Work out the finished part from the listing and answer in its coordinate system (mm). A direction names the side the tool comes from. Give positions to 0.01 mm unless a question says otherwise; leave off trailing zeros. Loops run counter-clockwise (first coordinate to the right, second up) from the corner with the lowest first, then second, coordinate; pieces in that order, holes last. Notation, with made-up numbers: (9, -25.75) - (36, -25.75) arc R25 ccw to (36, -12.75) - close; hole circle Ø11 at (-18.5, 69.5). An arc over 180 degrees is marked (long way). One line per question, with ' | ' between items. Start each with the question number.
1. Section C-C (y = 6.25) is taken. Determine the outline of the cut face in (x, z), plus the area to 3 significant figures.
2. Section B-B (x = 52) is taken. Determine the outline of the cut face in (y, z).
3. Find the intervals of material crossed by line 1 (Y direction, x = 34.5, z = 1.75); line 2 (X direction, y = 5, z = 12.75); line 3 (Y direction, x = 26.5, z = 7.5), in increasing order.
4. Which of the six approach directions +Z, -Z, +X, -X, +Y, -Y give full straight-line access (tool end or side, diameter ignored) to faces 1 (the face through (31, 21.971, 13)), 2 (the face through (1.651, 11, 6)), 3 (the face through (1.604, 20.45, 13.282)), 4 (the face through (31, 11.915, 5)), 5 (the face through (2.664, 11, 8))?
5. Each of these flat-tipped pins is pushed along its axis until it touches: pin 1 (3.5 mm diameter, centred on x = 34.5, z = 7.5, fed in from -Y); pin 2 (3 mm diameter, centred on y = 7, z = 9, fed in from -X); pin 3 (4 mm diameter, centred on x = 35, y = 11, fed in from +Z). Where does it stop, or does it pass through?
Autodesk Inventor part; units mm, degrees
ref_plane "YZ Plane" through (0, 0, 0) normal (1, 0, 0) x (0, 1, 0)
ref_plane "XZ Plane" through (0, 0, 0) normal (0, 1, 0) x (-1, 0, 0)
ref_plane "XY Plane" through (0, 0, 0) normal (0, 0, 1) x (1, 0, 0)
sketch "Sketch1" plane through (0, 0, 0) normal (0, 0, 1) x (1, 0, 0)
  line L0 (0, 0) -> (60.7568, 0)
  line L1 (60.7568, 0) -> (60.7568, 21.971)
  line L2 (60.7568, 21.971) -> (0, 21.971)
  line L3 (0, 21.971) -> (0, 0)
  dimension "d0" = 60.7568
  dimension "d1" = 21.971
extrude "Extrusion1" add sketch "Sketch1" along normal blind 14.1199
sketch "Sketch2" plane through (0, 0, 14.1199) normal (0, 0, 1) x (1, 0, 0)
  line L0 (0, 21.971) -> (60.7568, 21.971) construction
  line L1 (60.7568, 21.971) -> (60.7568, 0) construction
  line L2 (60.7568, 0) -> (0, 0) construction
  line L3 (0, 0) -> (0, 21.971) construction
  line L4 (58.0923, 19.3065) -> (2.6645, 19.3065)
  line L5 (2.6645, 19.3065) -> (2.6645, 2.6645)
  line L6 (2.6645, 2.6645) -> (58.0923, 2.6645)
  line L7 (58.0923, 2.6645) -> (58.0923, 19.3065)
  point P0 (0, 0)
  dimension "d4" = 2.6645
extrude "Extrusion2" cut sketch "Sketch2" against normal blind 12.319
sketch "Sketch3" plane through (0, 0, 0) normal (0, 0, -1) x (-1, 0, 0)
  line L0 (-60.7568, 21.971) -> (0, 21.971)
  line L1 (0, 21.971) -> (0, 0)
  line L2 (0, 0) -> (-60.7568, 0)
  line L3 (-60.7568, 0) -> (-60.7568, 21.971)
  line L4 (-1.651, 20.32) -> (-59.1058, 20.32)
  line L5 (-59.1058, 20.32) -> (-59.1058, 1.651)
  line L6 (-59.1058, 1.651) -> (-1.651, 1.651)
  line L7 (-1.651, 1.651) -> (-1.651, 20.32)
  dimension "d7" = 1.651
extrude "Extrusion3" cut sketch "Sketch3" against normal blind 12.4206
fillet "Fillet1" radius 5.334 8 edges at (0, 21.971, 13.2702) (60.7568, 21.971, 13.2702) (60.7568, 0, 13.2702) (0, 0, 13.2702) (1.651, 20.32, 6.2103) (59.1058, 20.32, 6.2103) (59.1058, 1.651, 6.2103) (1.651, 1.651, 6.2103)
sketch "Sketch4" plane through (0, 0, 1.8009) normal (0, 0, 1) x (1, 0, 0)
  line L0 (11.3005, 12.8295) -> (49.4563, 12.8295)
  line L1 (49.4563, 12.8295) -> (49.4563, 9.1415)
  line L2 (49.4563, 9.1415) -> (11.3005, 9.1415)
  line L3 (11.3005, 9.1415) -> (11.3005, 12.8295)
  line L4 (2.6645, 2.6645) -> (2.6645, 19.3065)
  line L5 (58.0923, 19.3065) -> (58.0923, 2.6645)
  line L6 (2.6645, 19.3065) -> (58.0923, 19.3065)
  line L7 (58.0923, 2.6645) -> (2.6645, 2.6645)
  line L8 (48.5419, 11.9151) -> (12.2149, 11.9151)
  line L9 (12.2149, 11.9151) -> (12.2149, 10.0559)
  line L10 (12.2149, 10.0559) -> (48.5419, 10.0559)
  line L11 (48.5419, 10.0559) -> (48.5419, 11.9151)
  point P0 (0, 0)
  dimension "d12" = 8.636
  dimension "d13" = 8.636
  dimension "d14" = 6.477
  dimension "d15" = 6.477
  dimension "d16" = 0.9144
extrude "Extrusion4" add sketch "Sketch4" along normal blind 6.223 contours L0 L1 L2 L3
sketch "Sketch5" plane through (0, 0, 1.8009) normal (0, 0, 1) x (1, 0, 0)
  line L0 (58.0923, 2.6645) -> (2.6645, 2.6645)
  line L1 (24.1275, 3.6297) -> (36.6293, 3.6297)
  line L2 (36.6293, 3.6297) -> (36.6293, 2.6645)
  line L3 (36.6293, 2.6645) -> (24.1275, 2.6645)
  line L4 (24.1275, 2.6645) -> (24.1275, 3.6297)
  line L5 (2.6645, 19.3065) -> (58.0923, 19.3065)
  line L6 (24.1275, 19.3065) -> (36.6293, 19.3065)
  line L7 (36.6293, 19.3065) -> (36.6293, 18.3413)
  line L8 (36.6293, 18.3413) -> (24.1275, 18.3413)
  line L9 (24.1275, 18.3413) -> (24.1275, 19.3065)
  line L10 (2.6645, 2.6645) -> (2.6645, 19.3065)
  line L11 (58.0923, 19.3065) -> (58.0923, 2.6645)
  point P0 (0, 0)
  dimension "d19" = 21.463
  dimension "d20" = 21.463
  dimension "d21" = 21.463
  dimension "d22" = 21.463
  dimension "d23" = 0.9652
  dimension "d24" = 0.9652
extrude "Extrusion5" cut sketch "Sketch5" against normal blind 6.223 contours L0 L4 L1 L2 | L7 L8 L9 L5
sketch "Sketch6" plane through (2.6645, 2.6645, 14.1199) normal (0, 1, 0) x (1, 0, 0)
  line L0 (55.4279, 0) -> (0, 0) construction
  line L1 (21.2344, 0) -> (34.1935, 0)
  line L2 (34.1935, 0) -> (34.1935, 0.9652)
  line L3 (34.1935, 0.9652) -> (21.2344, 0.9652)
  line L4 (21.2344, 0.9652) -> (21.2344, 0)
  line L5 (0, 0) -> (0, 12.319) construction
  line L6 (55.4279, 0) -> (55.4279, 12.319) construction
  point P0 (-2.6645, 14.1199)
  dimension "d27" = 21.2344
  dimension "d28" = 21.2344
  dimension "d29" = 0.9652
extrude "Extrusion6" add sketch "Sketch6" along normal up to next
sketch "Sketch7" plane through (0, 0, 14.1199) normal (0, 0, 1) x (1, 0, 0)
  line L0 (23.8989, 2.6645) -> (23.8989, 19.3065)
  line L1 (36.8579, 2.6645) -> (36.8579, 19.3065)
  line L2 (23.8989, 3.5789) -> (36.8579, 3.5789)
  line L3 (36.8579, 3.5789) -> (36.8579, 18.3921)
  line L4 (36.8579, 18.3921) -> (23.8989, 18.3921)
  line L5 (23.8989, 18.3921) -> (23.8989, 3.5789)
  line L6 (36.8579, 19.3065) -> (58.0923, 19.3065)
  line L7 (58.0923, 2.6645) -> (36.8579, 2.6645)
  point P0 (0, 0)
  dimension "d32" = 0.9144
  dimension "d33" = 0.9144
extrude "Extrusion7" cut sketch "Sketch7" against normal up to next
equation "\"d13\" = d12"
equation "\"d15\" = d14"
equation "\"d20\" = d19"
equation "\"d21\" = d19"
equation "\"d22\" = d20"
equation "\"d24\" = d23"
equation "\"d28\" = d27"
equation "\"d33\" = d32"
properties part number "Socket(ellipse Insert)"
Conclusion:
1) outline: (0, 12.42) - (1.7, 12.42) - (1.7, 0) - (59.05, 0) - (59.05, 12.42) - (60.76, 12.42) - (60.76, 14.12) - (58.09, 14.12) - (58.09, 1.8) - (2.66, 1.8) - (2.66, 14.12) - (0, 14.12) - close | area: 133 mm²
2) outline: (0, 12.42) - (1.65, 12.42) - (1.65, 0) - (20.32, 0) - (20.32, 12.42) - (21.97, 12.42) - (21.97, 14.12) - (19.31, 14.12) - (19.31, 1.8) - (2.66, 1.8) - (2.66, 14.12) - (0, 14.12) - close
3) line 1: 1.65 to 2.66, 3.63 to 18.34, 19.31 to 20.32 | line 2: 0.01 to 2.66, 58.09 to 60.75 | line 3: 1.65 to 2.66, 9.14 to 10.06, 11.92 to 12.83, 19.31 to 20.32
4) face 1: +Z, -Z, +X, -X, +Y | face 2: -Z, -X, +Y, -Y | face 3: +Z, -Z, -X, +Y | face 4: +Z | face 5: none
5) pin 1: y = 1.65 | pin 2: x = 1.65 | pin 3: z = 8.02
